Part model, mm, in its own coordinate system. A direction names the side the tool comes from. Coordinates: 2 decimals unless noted, no trailing zeros. Loops run counter-clockwise (first coordinate to the right, second up) from the corner with the lowest first, then second, coordinate; pieces in that order, holes last. Notation, with made-up numbers: M -7,57.5 L 24,57.5 A19 cw 24,87.5 Z; hole C 79,-30 d9. An arc over 180 degrees is marked long. Answer as CSV lines item,"result". Start each with the question number.
from build123d import *

# Parameters (mm, degrees)
SKETCH1_W            = 60
SKETCH1_H            = 127
BOSS_EXTRUDE1_DEPTH  = 1.5
CUT_EXTRUDE1_REACH   = 142.468
SKETCH2_R            = 1.5
BOSS_EXTRUDE2_DEPTH  = 3.5
BOSS_EXTRUDE3_DEPTH  = 4.8
BOSS_EXTRUDE4_DEPTH  = 1.2
SKETCH5_W            = 14.4
SKETCH5_H            = 2
BOSS_EXTRUDE5_DEPTH  = 14.5
BOSS_EXTRUDE6_DEPTH  = 1.4
BOSS_EXTRUDE7_DEPTH  = 7.6
SKETCH7_W            = 6.4
SKETCH7_H            = 5.3
BOSS_EXTRUDE8_DEPTH  = 15
SKETCH8_R            = 2.45
BOSS_EXTRUDE9_DEPTH  = 1
SKETCH5_2_W          = 14.4
SKETCH5_2_H          = 2
BOSS_EXTRUDE10_DEPTH = 0.25
SKETCH9_W            = 5.8
SKETCH9_H            = 12
BOSS_EXTRUDE11_DEPTH = 5.8


with BuildPart() as part:
    # Sketch1 → Boss-Extrude1 (new body)
    with BuildSketch(Plane(origin=(0, 0, 0), x_dir=(1, 0, 0), z_dir=(0, 1, 0))):
        with Locations((30, 63.5)):
            Rectangle(SKETCH1_W, SKETCH1_H)
    extrude(amount=BOSS_EXTRUDE1_DEPTH)

    # Sketch2 → Cut-Extrude1 (cut, up to next)
    with BuildSketch(Plane(origin=(0, 1.5, 0), x_dir=(1, 0, 0), z_dir=(0, 1, 0)), mode=Mode.PRIVATE) as cut_extrude1_sk1:
        with Locations(Location((4.19, 122.81, 0), (0, 0, 270))):
            Circle(SKETCH2_R)
    cut_extrude1_tool1 = extrude(cut_extrude1_sk1.sketch, amount=-CUT_EXTRUDE1_REACH, mode=Mode.PRIVATE) & part.part
    # Sketch2 → Cut-Extrude1 (cut, up to next)
    with BuildSketch(Plane(origin=(0, 1.5, 0), x_dir=(1, 0, 0), z_dir=(0, 1, 0)), mode=Mode.PRIVATE) as cut_extrude1_sk2:
        with Locations(Location((55.81, 122.81, 0), (0, 0, 270))):
            Circle(SKETCH2_R)
    cut_extrude1_tool2 = extrude(cut_extrude1_sk2.sketch, amount=-CUT_EXTRUDE1_REACH, mode=Mode.PRIVATE) & part.part
    # Sketch2 → Cut-Extrude1 (cut, up to next)
    with BuildSketch(Plane(origin=(0, 1.5, 0), x_dir=(1, 0, 0), z_dir=(0, 1, 0)), mode=Mode.PRIVATE) as cut_extrude1_sk3:
        with Locations(Location((4.19, 4.19, 0), (0, 0, 270))):
            Circle(SKETCH2_R)
    cut_extrude1_tool3 = extrude(cut_extrude1_sk3.sketch, amount=-CUT_EXTRUDE1_REACH, mode=Mode.PRIVATE) & part.part
    # Sketch2 → Cut-Extrude1 (cut, up to next)
    with BuildSketch(Plane(origin=(0, 1.5, 0), x_dir=(1, 0, 0), z_dir=(0, 1, 0)), mode=Mode.PRIVATE) as cut_extrude1_sk4:
        with Locations(Location((55.81, 4.19, 0), (0, 0, 270))):
            Circle(SKETCH2_R)
    cut_extrude1_tool4 = extrude(cut_extrude1_sk4.sketch, amount=-CUT_EXTRUDE1_REACH, mode=Mode.PRIVATE) & part.part
    add(cut_extrude1_tool1.solids().sort_by_distance((4.19, 1.5, -122.81))[0], mode=Mode.SUBTRACT)
    add(cut_extrude1_tool2.solids().sort_by_distance((55.81, 1.5, -122.81))[0], mode=Mode.SUBTRACT)
    add(cut_extrude1_tool3.solids().sort_by_distance((4.19, 1.5, -4.19))[0], mode=Mode.SUBTRACT)
    add(cut_extrude1_tool4.solids().sort_by_distance((55.81, 1.5, -4.19))[0], mode=Mode.SUBTRACT)

    # Sketch3 → Boss-Extrude2 (add)
    with BuildSketch(Plane(origin=(0, 1.5, 0), x_dir=(1, 0, 0), z_dir=(0, 1, 0))):
        with BuildLine():
            Line((5.324675365, 117), (54.675324635, 117))
            ThreePointArc((54.675324635, 117), (58.440438693, 115.440438693), (60, 111.675324635))
            Line((60, 111.675324635), (60, 15.324675365))
            ThreePointArc((60, 15.324675365), (58.440438693, 11.559561307), (54.675324635, 10))
            Line((54.675324635, 10), (5.324675365, 10))
            ThreePointArc((5.324675365, 10), (1.559561307, 11.559561307), (0, 15.324675365))
            Line((0, 15.324675365), (0, 111.675324635))
            ThreePointArc((0, 111.675324635), (1.559561307, 115.440438693), (5.324675365, 117))
        make_face()
    extrude(amount=BOSS_EXTRUDE2_DEPTH)



with BuildPart() as body_2:
    # Sketch4 → Boss-Extrude3 (new body)
    with BuildSketch(Plane.XY):
        with BuildLine():
            Line((18.35, 0), (25.65, 0))
            ThreePointArc((25.65, 0), (25.826776695, -0.073223305), (25.9, -0.25))
            Line((25.9, -0.25), (25.9, -2.25))
            ThreePointArc((25.9, -2.25), (25.826776695, -2.426776695), (25.65, -2.5))
            Line((25.65, -2.5), (18.35, -2.5))
            ThreePointArc((18.35, -2.5), (18.173223305, -2.426776695), (18.1, -2.25))
            Line((18.1, -2.25), (18.1, -0.25))
            ThreePointArc((18.1, -0.25), (18.173223305, -0.073223305), (18.35, 0))
        make_face()
    extrude(amount=-BOSS_EXTRUDE3_DEPTH)


with BuildPart() as part_1:
    add(part.part)

    add(body_2.part)  # Boss-Extrude4 merges body 2
    # Sketch4_2 → Boss-Extrude4 (add)
    with BuildSketch(Plane.XY):
        with BuildLine():
            Line((18.35, 0), (25.65, 0))
            ThreePointArc((25.65, 0), (25.826776695, -0.073223305), (25.9, -0.25))
            Line((25.9, -0.25), (25.9, -2.25))
            ThreePointArc((25.9, -2.25), (25.826776695, -2.426776695), (25.65, -2.5))
            Line((25.65, -2.5), (18.35, -2.5))
            ThreePointArc((18.35, -2.5), (18.173223305, -2.426776695), (18.1, -2.25))
            Line((18.1, -2.25), (18.1, -0.25))
            ThreePointArc((18.1, -0.25), (18.173223305, -0.073223305), (18.35, 0))
        make_face()
    extrude(amount=BOSS_EXTRUDE4_DEPTH)

    # Sketch5 → Boss-Extrude5 (add)
    with BuildSketch(Plane.ZY):
        with Locations((-35.3, -1)):
            Rectangle(SKETCH5_W, SKETCH5_H)
    extrude(amount=-BOSS_EXTRUDE5_DEPTH)



with BuildPart() as body_2_2:
    # Sketch6 → Boss-Extrude6 (new body)
    with BuildSketch(Plane(origin=(0, 0, -127), x_dir=(-1, 0, 0), z_dir=(0, 0, -1))):
        with BuildLine():
            Line((-28.308670428, 0), (-34.2, 0))
            ThreePointArc((-34.2, 0), (-34.376776695, -0.073223305), (-34.45, -0.25))
            Line((-34.45, -0.25), (-34.45, -1.65))
            ThreePointArc((-34.45, -1.65), (-34.523223305, -1.826776695), (-34.7, -1.9))
            Line((-34.7, -1.9), (-34.75, -1.9))
            ThreePointArc((-34.75, -1.9), (-34.926776695, -1.973223305), (-35, -2.15))
            Line((-35, -2.15), (-35, -3.55))
            ThreePointArc((-35, -3.55), (-34.926776695, -3.726776695), (-34.75, -3.8))
            Line((-34.75, -3.8), (-27.75, -3.8))
            ThreePointArc((-27.75, -3.8), (-27.573223305, -3.726776695), (-27.5, -3.55))
            Line((-27.5, -3.55), (-27.5, -2.15))
            ThreePointArc((-27.5, -2.15), (-27.573223305, -1.973223305), (-27.75, -1.9))
            Line((-27.75, -1.9), (-27.808670428, -1.9))
            ThreePointArc((-27.808670428, -1.9), (-27.985447123, -1.826776695), (-28.058670428, -1.65))
            Line((-28.058670428, -1.65), (-28.058670428, -0.25))
            ThreePointArc((-28.058670428, -0.25), (-28.131893732, -0.073223305), (-28.308670428, 0))
        make_face()
    extrude(amount=BOSS_EXTRUDE6_DEPTH)


with BuildPart() as part_2:
    add(part_1.part)

    add(body_2_2.part)  # Boss-Extrude7 merges body 2 2
    # Sketch6_3 → Boss-Extrude7 (add)
    with BuildSketch(Plane(origin=(0, 0, -127), x_dir=(-1, 0, 0), z_dir=(0, 0, -1))):
        with BuildLine():
            Line((-28.308670428, 0), (-34.2, 0))
            ThreePointArc((-34.2, 0), (-34.376776695, -0.073223305), (-34.45, -0.25))
            Line((-34.45, -0.25), (-34.45, -1.65))
            ThreePointArc((-34.45, -1.65), (-34.523223305, -1.826776695), (-34.7, -1.9))
            Line((-34.7, -1.9), (-34.75, -1.9))
            ThreePointArc((-34.75, -1.9), (-34.926776695, -1.973223305), (-35, -2.15))
            Line((-35, -2.15), (-35, -3.55))
            ThreePointArc((-35, -3.55), (-34.926776695, -3.726776695), (-34.75, -3.8))
            Line((-34.75, -3.8), (-27.75, -3.8))
            ThreePointArc((-27.75, -3.8), (-27.573223305, -3.726776695), (-27.5, -3.55))
            Line((-27.5, -3.55), (-27.5, -2.15))
            ThreePointArc((-27.5, -2.15), (-27.573223305, -1.973223305), (-27.75, -1.9))
            Line((-27.75, -1.9), (-27.808670428, -1.9))
            ThreePointArc((-27.808670428, -1.9), (-27.985447123, -1.826776695), (-28.058670428, -1.65))
            Line((-28.058670428, -1.65), (-28.058670428, -0.25))
            ThreePointArc((-28.058670428, -0.25), (-28.131893732, -0.073223305), (-28.308670428, 0))
        make_face()
    extrude(amount=-BOSS_EXTRUDE7_DEPTH)

    # Sketch7 → Boss-Extrude8 (add)
    with BuildSketch(Plane.ZY):
        with Locations((-102.7, -2.65)):
            Rectangle(SKETCH7_W, SKETCH7_H)
    extrude(amount=-BOSS_EXTRUDE8_DEPTH)

    # Sketch8 → Boss-Extrude9 (add)
    with BuildSketch(Plane.ZY):
        with Locations(Location((-102.7, -2.65, 0), (0, 0, 180))):
            Circle(SKETCH8_R)
    extrude(amount=BOSS_EXTRUDE9_DEPTH)

    # Sketch5_2 → Boss-Extrude10 (add)
    with BuildSketch(Plane.ZY):
        with Locations((-35.3, -1)):
            Rectangle(SKETCH5_2_W, SKETCH5_2_H)
    extrude(amount=BOSS_EXTRUDE10_DEPTH)

    # Sketch9 → Boss-Extrude11 (add)
    with BuildSketch(Plane(origin=(0, 0, -127), x_dir=(-1, 0, 0), z_dir=(0, 0, -1))):
        with Locations((-18.9, -6)):
            Rectangle(SKETCH9_W, SKETCH9_H)
    extrude(amount=-BOSS_EXTRUDE11_DEPTH)


solid = part_2.part
Q1. Slice it at A-A, the plane z = -122.81. State how many separate pieces and enclosed holes the cut face has, and give its area (3 significant figures).
Q2. Slice it at B-B, the plane y = 3. Write the cut outline in (x, z).
Q3. Flat gauge pins, fed straight in: P1, Ø2, axis at x = 22.5, y = -1.5, coming from the -Z side; P2, Ø1.8, axis at x = 23.5, z = -1.5, coming from the -Y side; P3, Ø2, axis at y = -1, z = -34.5, coming from the -X side. Where does each tip first touch, or does it go through?
Q4. Two-plate mould, pull along Z, no slides. Class faces 1 (the face through (-1, -3, -103)), 2 (the face through (58.4, 3.23, -115.48)), 3 (the face through (57.297, 0.76, -123.005)), 4 (the face through (5.455, 0.76, -122.004)): +Z half, -Z half, draft (parallel to the pull), parting line (faces both ways), or undercut.
Q5. Slice it at D-D, the plane z = -102.7. Write the cut outline in (x, y).
Q6. Wall check: L1, parallel to X at y = 0.75, z = -122.81; L2, parallel to Y at x = 37, z = -49; L3, parallel to Z at x = 3, y = -1.25. Give the ranges that are in metal, low to high.
Q7. Tool access for faces 5 (the face through (21.8, -6, -124)), 6 (the face through (7, -3, -99.5)), 7 (the face through (15, -3, -103)), 8 (the face through (19, -6, -121.2)), 9 (the face through (31, -2, -119.4)): list every direction of +Z, -Z, +X, -X, +Y, -Y with a clear straight run to the whole face (end or side of a thin tool).
Q8. Slice it at C-C, the plane z = -35.5. Write the cut outline in (x, y), and give its area (4 significant figures).
Solved:
1,separate pieces,"3"
1,enclosed holes,"0"
1,area,"177 mm2"
2,outline,"M 0,-111.68 A5.32 ccw 5.32,-117 L 54.68,-117 A5.32 ccw 60,-111.68 L 60,-15.32 A5.32 ccw 54.68,-10 L 5.32,-10 A5.32 ccw 0,-15.32 Z"
3,P1,"stops at z = -127"
3,P2,"stops at y = -2.5"
3,P3,"stops at x = -0.25"
4,face 1,"draft"
4,face 2,"-Z half"
4,face 3,"undercut"
4,face 4,"undercut"
5,outline,"M -1,-5.1 L 0,-5.1 L 0,-5.3 L 15,-5.3 L 15,0 L 60,0 L 60,5 L 0,5 L 0,-0.2 L -1,-0.2 Z"
6,L1,"x = 0 to 2.69, 5.69 to 54.31, 57.31 to 60"
6,L2,"y = 0 to 5"
6,L3,"z = -105.9 to -99.5, -42.5 to -28.1"
7,face 5,"-Z, -Y"
7,face 6,"+X, -X, -Y"
7,face 7,"+Z, -Z, +X, -Y"
7,face 8,"-X, -Y"
7,face 9,"+Z, +X, -X, -Y"
8,outline,"M -0.25,-2 L 14.5,-2 L 14.5,0 L 60,0 L 60,5 L 0,5 L 0,0 L -0.25,0 Z"
8,area,"329.5 mm2"
